```python
from build123d import *

# Parameters (mm, degrees)
F1_DEPTH = 25.4
F2_R     = 6.35
F3_DEPTH = 25.4
F5_DEPTH = 12.7


with BuildPart() as f1:
    # F0 (on Front) → F1 (new body)
    with BuildSketch(Plane.XZ):
        Polygon((0, 31.75), (0, 0), (69.85, 0), (69.85, 6.35), (25.4, 6.35), (25.4, 31.75), align=None)
    extrude(amount=F1_DEPTH)

    # F2 (on face) → F3 (cut)
    with BuildSketch(Plane.XZ.offset(25.4)):
        with BuildLine():
            ThreePointArc((0, 19.05), (3.719744, 28.030256), (12.7, 31.75))
            Line((12.7, 31.75), (0, 31.75))
            Line((0, 31.75), (0, 19.05))
        make_face()
        with BuildLine():
            ThreePointArc((12.7, 31.75), (21.680256, 28.030256), (25.4, 19.05))
            Line((25.4, 19.05), (25.4, 31.75))
            Line((25.4, 31.75), (12.7, 31.75))
        make_face()
        with Locations((12.7, 19.05)):
            Circle(F2_R)
    extrude(amount=-F3_DEPTH, mode=Mode.SUBTRACT)

    # F4 (on face) → F5 (cut)
    with BuildSketch(Plane.XY.offset(6.35)):
        with BuildLine():
            Line((38.1, -12.7), (38.1, -6.35))
            ThreePointArc((38.1, -6.35), (31.75, -12.7), (38.1, -19.05))
            Line((38.1, -19.05), (38.1, -12.7))
        make_face()
        with BuildLine():
            ThreePointArc((44.45, -12.7), (42.590128, -8.209872), (38.1, -6.35))
            Line((38.1, -6.35), (38.1, -12.7))
            Line((38.1, -12.7), (38.1, -19.05))
            ThreePointArc((38.1, -19.05), (42.590128, -17.190128), (44.45, -12.7))
        make_face()
        with BuildLine():
            ThreePointArc((57.15, -19.05), (50.8, -12.7), (57.15, -6.35))
            Line((57.15, -6.35), (38.1, -6.35))
            ThreePointArc((38.1, -6.35), (42.590128, -8.209872), (44.45, -12.7))
            ThreePointArc((44.45, -12.7), (42.590128, -17.190128), (38.1, -19.05))
            Line((38.1, -19.05), (57.15, -19.05))
        make_face()
        with BuildLine():
            ThreePointArc((57.15, 0), (66.130256, -3.719744), (69.85, -12.7))
            Line((69.85, -12.7), (69.85, 0))
            Line((69.85, 0), (57.15, 0))
        make_face()
        with BuildLine():
            ThreePointArc((69.85, -12.7), (66.130256, -21.680256), (57.15, -25.4))
            Line((57.15, -25.4), (69.85, -25.4))
            Line((69.85, -25.4), (69.85, -12.7))
        make_face()
        with BuildLine():
            ThreePointArc((57.15, -19.05), (61.640128, -17.190128), (63.5, -12.7))
            ThreePointArc((63.5, -12.7), (61.640128, -8.209872), (57.15, -6.35))
            Line((57.15, -6.35), (57.15, -19.05))
        make_face()
        with BuildLine():
            Line((57.15, -19.05), (57.15, -6.35))
            ThreePointArc((57.15, -6.35), (50.8, -12.7), (57.15, -19.05))
        make_face()
    extrude(amount=-F5_DEPTH, mode=Mode.SUBTRACT)


solid = f1.part
```
CAD build for the part. Positions are in the model's coordinates, mm. A direction names the side the tool comes from. Round coordinates to 2 decimals unless told otherwise and drop trailing zeros. Loops run counter-clockwise (first coordinate to the right, second up) from the corner with the lowest first, then second, coordinate; pieces in that order, holes last. Notation, with made-up numbers: (13.5, -36.5) - (52.5, -36.5) arc R36 ccw to (52.5, -1.5) - close; hole circle Ø2 at (40.5, 87). An arc over 180 degrees is marked (long way). Return JSON: item names as keys, results as strings. Group by question number.
Q1. Two-plate mould, pull along X, no slides. Class faces 1 (the face through (0, -13, 10)), 2 (the face through (25.4, -13, 13)), 3 (the face through (47, -19.05, 3)), 4 (the face through (22, -25.4, 13)): +X half, -X half, draft (parallel to the pull), parting line (faces both ways), or undercut.
Q2. Flat gauge pins, fed straight in: pin 1 Ø1 at (y, z) = (-12.5, 15.5) entering from +X; pin 2 Ø2 at (y, z) = (-19, 4) entering from +X; pin 3 Ø5 at (x, y) = (25, -15.5) entering from -Z. Where does each tip first touch, or does it go through?
Q3. Band-saw the part on D-D on z = 14. Give the cut face in (x, y).
Q4. Drill centre lines: line 1 along Z through (x, y) = (12.7, -13); line 2 along X through (y, z) = (-8.75, 6); line 3 along Z through (x, y) = (30, -17.5). Where is each one in solid material? Low to high. Write a range as [from, to].
Q5. Band-saw the part on C-C on z = 5.5. Give the cut face in (x, y), plus the area to 3 significant figures.
Q6. Band-saw the part on B-B on y = -10.5. Give the cut face in (x, z), plus the area to 3 significant figures.
Q7. Band-saw the part on A-A on x = 51.5. Give the cut face in (y, z), plus the area to 3 significant figures.
Q8. Tool access for faces 5 (the face through (48, -21, 6.35)), 6 (the face through (27, -13, 0)), 7 (the face through (48, -6.35, 3)): list every direction of +Z, -Z, +X, -X, +Y, -Y with a clear straight run to the whole face (end or side of a thin tool).
Solutions:
{
 "1": {"face 1": "-X half", "face 2": "+X half", "face 3": "undercut", "face 4": "draft"},
 "2": {"pin 1": "stops at x = 25.4", "pin 2": "stops at x = 68.69", "pin 3": "stops at z = 0"},
 "3": {"outline": "(0, -25.4) - (8.85, -25.4) - (8.85, 0) - (0, 0) - close; (16.55, -25.4) - (25.4, -25.4) - (25.4, 0) - (16.55, 0) - close"},
 "4": {"line 1": "z = [0, 12.7], [25.4, 31.75]", "line 2": "x = [0, 33.13], [62.12, 69.22]", "line 3": "z = [0, 6.35]"},
 "5": {"outline": "(0, -25.4) - (57.15, -25.4) arc R12.7 ccw to (57.15, 0) - (0, 0) - close; hole (38.1, -19.05) - (57.15, -19.05) arc R6.35 ccw to (57.15, -6.35) - (38.1, -6.35) arc R6.35 ccw to start", "area": "1,340 mm^2"},
 "6": {"outline": "(0, 0) - (32.14, 0) - (32.14, 6.35) - (25.4, 6.35) - (25.4, 19.05) arc R12.7 ccw to (0, 19.05) - close; (63.11, 0) - (69.66, 0) - (69.66, 6.35) - (63.11, 6.35) - close; hole circle Ø12.7 at (12.7, 19.05)", "area": "695 mm^2"},
 "7": {"outline": "(-25.4, 0) - (-19.05, 0) - (-19.05, 6.35) - (-25.4, 6.35) - close; (-6.35, 0) - (0, 0) - (0, 6.35) - (-6.35, 6.35) - close", "area": "80.6 mm^2"},
 "8": {"face 5": "+Z, +X, +Y, -Y", "face 6": "-Z, +X, -X, +Y, -Y", "face 7": "+Z, -Z"}
}
